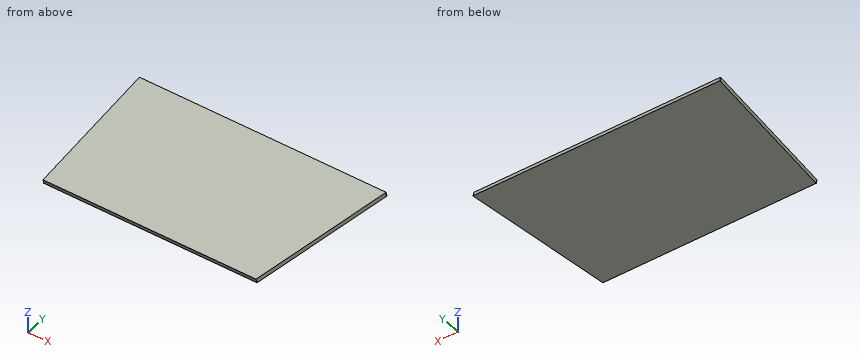
from build123d import *

# Parameters (mm, degrees)
BOSS_EXTRU_1_DEPTH           = 30
BOSS_EXTRU_2_DEPTH           = 970.2413
BOSS_EXTRU_2_DEPTH_BACK      = 715.8287
ENL_V_MAT_EXTRU_1_DEPTH      = 970.2413
ENL_V_MAT_EXTRU_1_DEPTH_BACK = 970.2413


with BuildPart() as part:
    # Esquisse1 → Boss.-Extru.1 (new body)
    with BuildSketch(Plane.XY):
        Polygon((-715.828706454, 477.703685082), (970.241293546, 477.703685082), (855.251293546, -558.817416632), (-600.838706454, -558.817416632), align=None)
    extrude(amount=BOSS_EXTRU_1_DEPTH)

    # Esquisse2 → Boss.-Extru.2 (add, two sides: drawn at the far end of the back side and taken through both)
    with BuildSketch(Plane(origin=(0, 0, 0), x_dir=(0, 0, -1), z_dir=(1, 0, 0)).offset(-BOSS_EXTRU_2_DEPTH_BACK)):
        Polygon((-30, 477.703685082), (0, 477.703685082), (0, 485.832018962), align=None)
    extrude(amount=BOSS_EXTRU_2_DEPTH + BOSS_EXTRU_2_DEPTH_BACK)

    # Esquisse3 → Enlèv. mat.-Extru.1 (cut, two sides: drawn at the far end of the back side and taken through both)
    with BuildSketch(Plane(origin=(0, 0, 0), x_dir=(0, 0, -1), z_dir=(1, 0, 0)).offset(-ENL_V_MAT_EXTRU_1_DEPTH_BACK)):
        Polygon((-30, -558.817416632), (0, -550.689082753), (0, -558.817416632), align=None)
    extrude(amount=ENL_V_MAT_EXTRU_1_DEPTH + ENL_V_MAT_EXTRU_1_DEPTH_BACK, mode=Mode.SUBTRACT)


solid = part.part
Input: part model. Units: mm. Frame: model coordinates. Round coordinates to 2 decimals unless told otherwise and drop trailing zeros. Order: outer loops, then holes, each group sorted by start corner. A loop starts at its lowest first (then second) coordinate and runs counter-clockwise, first axis right, second up.
1. Cut plane C-C, the plane y = -183. Output: boundary loops of the cut face in (x, z).
The answers:
outline: (-642.53, 0) - (896.94, 0) - (896.94, 30) - (-642.53, 30) - close
2. Material intervals for line 1 (X direction, y = -455, z = 26); line 2 (X direction, y = 42, z = 12.5); line 3 (Y direction, x = -387, z = 7.5), sorted ascending.
The answers:
line 1: x = -612.36 to 866.77
line 2: x = -667.49 to 921.91
line 3: y = -552.72 to 483.8
3. Cut plane B-B, the plane y = 174. Output: boundary loops of the cut face in (x, z), then the cut area to 3 significant figures.
The answers:
outline: (-682.14, 0) - (936.55, 0) - (936.55, 30) - (-682.14, 30) - close
area: 48,600 mm2
4. Pin query (flat end, axial travel): P1, Ø8, axis at x = 727, z = 24.5, coming from the +Y side; P2, Ø12, axis at x = -36, z = 14.5, coming from the +Y side; P3, Ø8, axis at y = -122.5, z = 7, coming from the -X side. Return the tip coordinate at first contact, or that it passes through.
The answers:
P1: stops at y = 480.28
P2: stops at y = 483.53
P3: stops at x = -649.69
